```python
from build123d import *

# Parameters (mm, degrees)
PAD_DEPTH   = 50
THICKNESS_T = 1.5


with BuildPart() as part:
    # Sketch → Pad (new body)
    with BuildSketch(Plane.XY):
        with BuildLine():
            ThreePointArc((3, 0), (0.87868, -0.87868), (0, -3))
            Line((0, -50), (0, -3))
            ThreePointArc((0, -50), (0.87868, -52.12132), (3, -53))
            Line((75, -53), (3, -53))
            ThreePointArc((75, -53), (77.12132, -52.12132), (78, -50))
            Line((78, -3), (78, -50))
            ThreePointArc((78, -3), (77.12132, -0.87868), (75, 0))
            Line((3, 0), (75, 0))
        make_face()
    extrude(amount=PAD_DEPTH)

    # Thickness
    thickness_openings = [part.faces().sort_by_distance(p)[0] for p in [
        (39, -26.5, 50),
    ]]
    offset(amount=THICKNESS_T, openings=thickness_openings)


solid = part.part
```
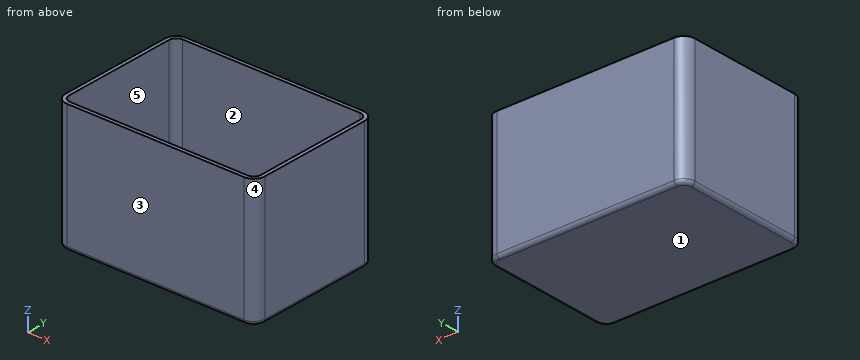
Check sheet for the modelled part. Datum: model origin and axes. Units: mm. Face numbers are marked on the shaded views. A direction names the side the tool comes from. Give positions to 0.01 mm unless a question says otherwise; leave off trailing zeros. Write each loop counter-clockwise with the first axis right and the second up, starting at its lowest first coordinate (ties: lowest second). Pieces come first, ordered by that corner, then holes.
Item 1: Cross-section at A-A (y = -5.5). Enter the section's corners in (x, z), and give its area (3 significant figures).
Item 2: Scan lines: L1, parallel to X at y = -49.5, z = 31.5; L2, parallel to Y at x = 46, z = 22; L3, parallel to Z at x = 54.5, y = -33. Record each from-to range of solid material in increasing order.
Item 3: Draft check along Y on the marked faces 1, 2 and 3. Enter one of: released by +Y, released by -Y, zero draft, split by the parting line, or undercut.
Item 4: Access from +Z, -Z, +X, -X, +Y, -Y to the whole of each face (thin tool, end or side, straight path). Record for the marked faces 4 and 5.
Item 5: Gauge pin test, flat end, axial feed: pin 1 (2 mm diameter, centred on x = 50.5, y = -20.5, fed in from +Z). Record the tip position at first contact, or that the pin passes through.
Item 6: Cross-section at B-B (z = 35). Enter the section's corners in (x, y), and give its area (3 significant figures).
Item 7: Cross-section at C-C (x = 65.5). Enter the section's corners in (y, z), and give its area (3 significant figures).
Report:
1. outline: (-1.5, 0) arc R1.5 ccw to (0, -1.5) - (78, -1.5) arc R1.5 ccw to (79.5, 0) - (79.5, 50) - (78, 50) - (78, 0) - (0, 0) - (0, 50) - (-1.5, 50) - close
1. area: 271 mm2
2. L1: x = -1.5 to 0, 78 to 79.5
2. L2: y = -54.5 to -53, 0 to 1.5
2. L3: z = -1.5 to 0
3. face 1: zero draft
3. face 2: undercut
3. face 3: released by -Y
4. face 4: +Z, -Z, +X, -Y
4. face 5: +Z
5. pin 1: stops at z = 0
6. outline: (-1.5, -50) arc R4.5 ccw to (3, -54.5) - (75, -54.5) arc R4.5 ccw to (79.5, -50) - (79.5, -3) arc R4.5 ccw to (75, 1.5) - (3, 1.5) arc R4.5 ccw to (-1.5, -3) - close; hole (0, -50) arc R3 ccw to (3, -53) - (75, -53) arc R3 ccw to (78, -50) - (78, -3) arc R3 ccw to (75, 0) - (3, 0) arc R3 ccw to (0, -3) - close
6. area: 392 mm2
7. outline: (-54.5, 0) arc R1.5 ccw to (-53, -1.5) - (0, -1.5) arc R1.5 ccw to (1.5, 0) - (1.5, 50) - (0, 50) - (0, 0) - (-53, 0) - (-53, 50) - (-54.5, 50) - close
7. area: 233 mm2
